Geometry check sheet. Reference: the model listing, model coordinates, mm. Give positions to 0.01 mm unless a question says otherwise; leave off trailing zeros. Write each loop counter-clockwise with the first axis right and the second up, starting at its lowest first coordinate (ties: lowest second). Pieces come first, ordered by that corner, then holes.
(1) Cross-section at A-A (y = 18.5). Record the boundary of the cut face in (x, z).
(2) Mould release check, pull along X, two halves, no side actions. Record for faces 1 (the cylindrical face through (-17.342, 20.924, 1.528)), 2 (the flat face through (0, -11, 3.1)): +X half, -X half, draft (parallel to the pull), parting line (faces both ways), or undercut.
(3) Cross-section at B-B (z = 1.45). Count the separate pieces of the cut face and the enclosed holes in it, and give its area (3 significant figures).
(4) Thickness scan on line 1 along Y through (x, z) = (15, 2.6); line 2 along Y through (x, z) = (-2, 0.35); line 3 along Y through (x, z) = (-9, 2.4). Record the ranges inside material, lowest first.
(5) Depth check by flat-ended pin: P1, Ø10, axis at x = -6.86, y = -18.85, coming from the -Z side; P2, Ø8, axis at x = -19.76, y = 3.48, coming from the -Z side; P3, Ø1, axis at x = 20, z = 2, coming from the +Y side. Enter the tip coordinate at first touch or a pass-through.
```python
from build123d import *

# Parameters (mm, degrees)
F0_R     = 4.4
F1_DEPTH = 3.1


with BuildPart() as f1:
    # F0 (on Top) → F1 (new body)
    with BuildSketch(Plane.XY):
        with BuildLine():
            ThreePointArc((20.42269, -3.601071), (26.764785, 4.719354), (17.959412, 10.368871))
            ThreePointArc((17.959412, 10.368871), (17.469473, 20.819307), (7.092726, 19.487104))
            ThreePointArc((7.092726, 19.487104), (0, 27.177675), (-7.092726, 19.487104))
            ThreePointArc((-7.092726, 19.487104), (-17.469473, 20.819307), (-17.959412, 10.368871))
            ThreePointArc((-17.959412, 10.368871), (-26.764785, 4.719354), (-20.42269, -3.601071))
            ThreePointArc((-20.42269, -3.601071), (-23.536557, -13.588838), (-13.329964, -15.886033))
            ThreePointArc((-13.329964, -15.886033), (-9.295312, -25.538661), (0, -20.737743))
            ThreePointArc((0, -20.737743), (9.295312, -25.538661), (13.329964, -15.886033))
            ThreePointArc((13.329964, -15.886033), (23.536557, -13.588838), (20.42269, -3.601071))
        make_face()
        with Locations((-6.86151, -18.851843)):
            Circle(F0_R, mode=Mode.SUBTRACT)
        with BuildLine():
            ThreePointArc((0, -16.965943), (-0.69539, -15.299956), (-1.787641, -13.862575))
            ThreePointArc((-1.787641, -13.862575), (-0.895661, -13.948635), (0, -13.977362))
            ThreePointArc((0, -13.977362), (0.895661, -13.948635), (1.787641, -13.862575))
            ThreePointArc((1.787641, -13.862575), (0.69539, -15.299956), (0, -16.965943))
        make_face(mode=Mode.SUBTRACT)
        with Locations((-17.373952, -10.030856)):
            Circle(F0_R, mode=Mode.SUBTRACT)
        with BuildLine():
            ThreePointArc((-16.708192, -2.946105), (-15.188268, -1.971984), (-13.962392, -0.646728))
            ThreePointArc((-13.962392, -0.646728), (-13.892254, -1.540101), (-13.765014, -2.427143))
            ThreePointArc((-13.765014, -2.427143), (-13.581194, -3.304209), (-13.34155, -4.167694))
            ThreePointArc((-13.34155, -4.167694), (-14.946762, -3.341635), (-16.708192, -2.946105))
        make_face(mode=Mode.SUBTRACT)
        with BuildLine():
            ThreePointArc((-10.905498, -12.996666), (-10.367322, -11.273458), (-10.280104, -9.470275))
            ThreePointArc((-10.280104, -9.470275), (-9.652127, -10.109555), (-8.984475, -10.70728))
            ThreePointArc((-8.984475, -10.70728), (-8.279894, -11.260995), (-7.541278, -11.768422))
            ThreePointArc((-7.541278, -11.768422), (-9.301923, -12.167434), (-10.905498, -12.996666))
        make_face(mode=Mode.SUBTRACT)
        with BuildLine():
            ThreePointArc((-3.595662, 9.878999), (0, 10.513011), (3.595662, 9.878999))
            ThreePointArc((3.595662, 9.878999), (6.757633, 8.053434), (9.104535, 5.256506))
            ThreePointArc((9.104535, 5.256506), (10.353295, 1.825565), (10.353295, -1.825565))
            ThreePointArc((10.353295, -1.825565), (9.104535, -5.256506), (6.757633, -8.053434))
            ThreePointArc((6.757633, -8.053434), (3.595662, -9.878999), (0, -10.513011))
            ThreePointArc((0, -10.513011), (-3.595662, -9.878999), (-6.757633, -8.053434))
            ThreePointArc((-6.757633, -8.053434), (-9.104535, -5.256506), (-10.353295, -1.825565))
            ThreePointArc((-10.353295, -1.825565), (-10.353295, 1.825565), (-9.104535, 5.256506))
            ThreePointArc((-9.104535, 5.256506), (-6.757633, 8.053434), (-3.595662, 9.878999))
        make_face(mode=Mode.SUBTRACT)
        with Locations((6.86151, -18.851843)):
            Circle(F0_R, mode=Mode.SUBTRACT)
        with BuildLine():
            ThreePointArc((10.905498, -12.996666), (9.301923, -12.167434), (7.541278, -11.768422))
            ThreePointArc((7.541278, -11.768422), (8.279894, -11.260995), (8.984475, -10.70728))
            ThreePointArc((8.984475, -10.70728), (9.652127, -10.109555), (10.280104, -9.470275))
            ThreePointArc((10.280104, -9.470275), (10.367322, -11.273458), (10.905498, -12.996666))
        make_face(mode=Mode.SUBTRACT)
        with Locations((17.373952, -10.030856)):
            Circle(F0_R, mode=Mode.SUBTRACT)
        with BuildLine():
            ThreePointArc((16.708192, -2.946105), (14.946762, -3.341635), (13.34155, -4.167694))
            ThreePointArc((13.34155, -4.167694), (13.581194, -3.304209), (13.765014, -2.427143))
            ThreePointArc((13.765014, -2.427143), (13.892254, -1.540101), (13.962392, -0.646728))
            ThreePointArc((13.962392, -0.646728), (15.188268, -1.971984), (16.708192, -2.946105))
        make_face(mode=Mode.SUBTRACT)
        with Locations((-19.756929, 3.48368)):
            Circle(F0_R, mode=Mode.SUBTRACT)
        with BuildLine():
            ThreePointArc((-14.692937, 8.482971), (-12.902456, 8.252203), (-11.111521, 8.47943))
            ThreePointArc((-11.111521, 8.47943), (-11.632042, 7.749983), (-12.10475, 6.988681))
            ThreePointArc((-12.10475, 6.988681), (-12.527703, 6.198652), (-12.899163, 5.383144))
            ThreePointArc((-12.899163, 5.383144), (-13.597845, 7.047753), (-14.692937, 8.482971))
        make_face(mode=Mode.SUBTRACT)
        with Locations((-12.89542, 15.368163)):
            Circle(F0_R, mode=Mode.SUBTRACT)
        with BuildLine():
            ThreePointArc((-5.802694, 15.942771), (-4.57944, 14.615093), (-3.061446, 13.637969))
            ThreePointArc((-3.061446, 13.637969), (-3.929068, 13.413764), (-4.780539, 13.134424))
            ThreePointArc((-4.780539, 13.134424), (-5.612361, 12.801095), (-6.421113, 12.41515))
            ThreePointArc((-6.421113, 12.41515), (-5.886346, 14.139418), (-5.802694, 15.942771))
        make_face(mode=Mode.SUBTRACT)
        with Locations((0, 20.061712)):
            Circle(F0_R, mode=Mode.SUBTRACT)
        with BuildLine():
            ThreePointArc((14.692937, 8.482971), (13.597845, 7.047753), (12.899163, 5.383144))
            ThreePointArc((12.899163, 5.383144), (12.527703, 6.198652), (12.10475, 6.988681))
            ThreePointArc((12.10475, 6.988681), (11.632042, 7.749983), (11.111521, 8.47943))
            ThreePointArc((11.111521, 8.47943), (12.902456, 8.252203), (14.692937, 8.482971))
        make_face(mode=Mode.SUBTRACT)
        with Locations((19.756929, 3.48368)):
            Circle(F0_R, mode=Mode.SUBTRACT)
        with BuildLine():
            ThreePointArc((4.780539, 13.134424), (3.929068, 13.413764), (3.061446, 13.637969))
            ThreePointArc((3.061446, 13.637969), (4.57944, 14.615093), (5.802694, 15.942771))
            ThreePointArc((5.802694, 15.942771), (5.886346, 14.139418), (6.421113, 12.41515))
            ThreePointArc((6.421113, 12.41515), (5.612361, 12.801095), (4.780539, 13.134424))
        make_face(mode=Mode.SUBTRACT)
        with Locations((12.89542, 15.368163)):
            Circle(F0_R, mode=Mode.SUBTRACT)
    extrude(amount=F1_DEPTH)


solid = f1.part
```
Reply:
1. outline: (-19.29, 0) - (-15.99, 0) - (-15.99, 3.1) - (-19.29, 3.1) - close; (-9.8, 0) - (-4.11, 0) - (-4.11, 3.1) - (-9.8, 3.1) - close; (4.11, 0) - (9.8, 0) - (9.8, 3.1) - (4.11, 3.1) - close; (15.99, 0) - (19.29, 0) - (19.29, 3.1) - (15.99, 3.1) - close
2. face 1: undercut
2. face 2: draft
3. separate pieces: 1
3. enclosed holes: 19
3. area: 1,100 mm2
4. line 1: y = -16.74 to -13.74, -6.33 to -3.32, -1.81 to 11.5, 19.23 to 22.17
4. line 2: y = -24.05 to -10.32, 10.32 to 16.14, 23.98 to 26.89
4. line 3: y = -25.64 to -22.7, -15.01 to -12.06, -10.69 to -5.43, 5.43 to 13.32, 17.41 to 21.32
5. P1: stops at z = 0
5. P2: passes through
5. P3: stops at y = 18.02
